from build123d import *

# Parameters (mm, degrees)
BOSS_EXTRUDE1_DEPTH = 5
SKETCH2_R           = 1.7
SKETCH2_W           = 8.5
SKETCH2_H           = 13.5
CUT_EXTRUDE2_DEPTH  = 5


with BuildPart() as part:
    # Sketch1 → Boss-Extrude1 (new body)
    with BuildSketch(Plane.XY):
        with BuildLine():
            Line((-55, 43), (55, 43))
            ThreePointArc((55, 43), (62.071067812, 40.071067812), (65, 33))
            Line((65, 33), (65, -33))
            ThreePointArc((65, -33), (62.071067812, -40.071067812), (55, -43))
            Line((55, -43), (-55, -43))
            ThreePointArc((-55, -43), (-62.071067812, -40.071067812), (-65, -33))
            Line((-65, -33), (-65, 33))
            ThreePointArc((-65, 33), (-62.071067812, 40.071067812), (-55, 43))
        make_face()
    extrude(amount=BOSS_EXTRUDE1_DEPTH)

    # Sketch2 → Cut-Extrude2 (cut)
    with BuildSketch(Plane.XY.offset(5)):
        with Locations((-52, 23)):
            Circle(SKETCH2_R)
        with Locations((-52, -23)):
            Circle(SKETCH2_R)
        with Locations((52, -23)):
            Circle(SKETCH2_R)
        with Locations((52, 23)):
            Circle(SKETCH2_R)
        with Locations((-41.25, -15.05)):
            Circle(SKETCH2_R)
        with Locations((-41.25, 15.075)):
            Circle(SKETCH2_R)
        with Locations((41.25, -15.05)):
            Circle(SKETCH2_R)
        with Locations((41.25, 15.075)):
            Circle(SKETCH2_R)
        with BuildLine():
            Line((-15, -28), (15, -28))
            ThreePointArc((15, -28), (20, -33), (15, -38))
            Line((15, -38), (-15, -38))
            ThreePointArc((-15, -38), (-20, -33), (-15, -28))
        make_face()
        with BuildLine():
            Line((-15, 38), (15, 38))
            ThreePointArc((15, 38), (20, 33), (15, 28))
            Line((15, 28), (-15, 28))
            ThreePointArc((-15, 28), (-20, 33), (-15, 38))
        make_face()
        with Locations((55, 0)):
            Rectangle(SKETCH2_W, SKETCH2_H)
    extrude(amount=-CUT_EXTRUDE2_DEPTH, mode=Mode.SUBTRACT)


solid = part.part
Source: CAD feature listing. Evaluate the final solid. Frame: model axes, mm. A direction names the side the tool comes from. Coordinates: 2 decimals unless noted, no trailing zeros. Write each loop counter-clockwise with the first axis right and the second up, starting at its lowest first coordinate (ties: lowest second). Pieces come first, ordered by that corner, then holes. Notation, with made-up numbers: M 67.5,42.25 L 113.5,42.25 A33 ccw 113.5,75.25 Z; hole C 65.5,37.5 d5. An arc over 180 degrees is marked long. Use a Markdown table: item, result.
1) Mould query, pull axis Y, two halves, no side actions, for faces 1 (the cylindrical face through (50.3, -22.93, 2.54)), 2 (the flat face through (1, -43, 2)), 3 (the flat face through (1, 1, 5)), 4 (the cylindrical face through (39.997, 16.224, 2.535)). Classes: pulls with the +Y half, pulls with the -Y half, needs draft (parallel to the pull), parting line crosses it, or undercut.
Conclusion:
| item | result |
|---|---|
| face 1 | undercut |
| face 2 | pulls with the -Y half |
| face 3 | needs draft |
| face 4 | undercut |
2) Section B-B, the plane y = -23. Output: boundary loops of the cut face in (x, z), then the cut area to 3 significant figures.
Conclusion:
| item | result |
|---|---|
| outline | M -65,0 L -53.7,0 L -53.7,5 L -65,5 Z; M -50.3,0 L 50.3,0 L 50.3,5 L -50.3,5 Z; M 53.7,0 L 65,0 L 65,5 L 53.7,5 Z |
| area | 616 mm^2 |
3) Section A-A, the plane x = -52. Output: boundary loops of the cut face in (y, z).
Conclusion:
| item | result |
|---|---|
| outline | M -43,0 L -24.7,0 L -24.7,5 L -43,5 Z; M -21.3,0 L 21.3,0 L 21.3,5 L -21.3,5 Z; M 24.7,0 L 43,0 L 43,5 L 24.7,5 Z |
4) Reachability of faces 5 (the cylindrical face through (61.99, 40.15, 2.46)), 6 (the flat face through (0, -28, 3)) from +Z, -Z, +X, -X, +Y, -Y: full face, straight path, thin tool, end or side. Return the list, or none.
Conclusion:
| item | result |
|---|---|
| face 5 | +Z, -Z, +X, +Y |
| face 6 | +Z, -Z |
5) Section C-C, the plane z = 4.05. Give the number of separate pieces and of enclosed holes in the cut face, then the cut area to 3 significant figures.
Conclusion:
| item | result |
|---|---|
| separate pieces | 1 |
| enclosed holes | 11 |
| area | 10,100 mm^2 |
6) Ray query, L1, parallel to Y at x = 52, z = 1.75; L2, parallel to Y at x = 14, z = 3.15; L3, parallel to Y at x = 41.25, z = 2 (3 decimals). Return the intervals inside material, ascending.
Conclusion:
| item | result |
|---|---|
| L1 | y = -43 to -24.7, -21.3 to -6.75, 6.75 to 21.3, 24.7 to 43 |
| L2 | y = -43 to -38, -28 to 28, 38 to 43 |
| L3 | y = -43 to -16.75, -13.35 to 13.375, 16.775 to 43 |
